Geometry check sheet. Reference: the model listing, model coordinates, mm. Face numbers are marked on the shaded views. A direction names the side the tool comes from. Give positions to 0.01 mm unless a question says otherwise; leave off trailing zeros. Order: outer loops, then holes, each group sorted by start corner. A loop starts at its lowest first (then second) coordinate and runs counter-clockwise, first axis right, second up.
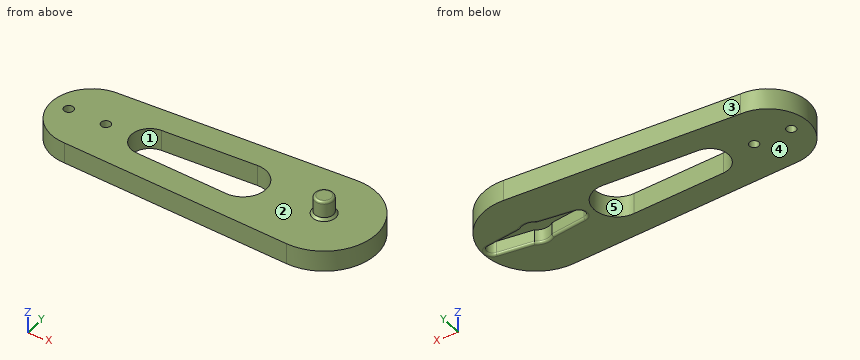
```python
from build123d import *

# Parameters (mm, degrees)
BOSS_EXTRUDE1_DEPTH = 9
BOSS_EXTRUDE2_START = 9
SKETCH3_R           = 4
BOSS_EXTRUDE2_DEPTH = 8
FILLET1_R           = 1
CHAMFER2_SIZE       = 1
CUT_EXTRUDE1_DEPTH  = 6
FILLET3_R           = 1
SKETCH6_R           = 2.05
CUT_EXTRUDE2_DEPTH  = 10


with BuildPart() as part:
    # Sketch2 → Boss-Extrude1 (new body)
    with BuildSketch(Plane(origin=(0, 0, 0), x_dir=(0, 1, 0), z_dir=(0, 0, 1))):
        with BuildLine():
            Line((22.471608109, 1.129968581), (17.5, 100))
            ThreePointArc((17.5, 100), (0, 117.5), (-17.5, 100))
            Line((-17.5, 100), (-22.471608109, 1.129968581))
            ThreePointArc((-22.471608109, 1.129968581), (0, -22.5), (22.471608109, 1.129968581))
        make_face()
    extrude(amount=BOSS_EXTRUDE1_DEPTH)

    # Sketch3 → Boss-Extrude2 (add)
    with BuildSketch(Plane(origin=(0, 0, 0), x_dir=(0, 1, 0), z_dir=(0, 0, 1)).offset(BOSS_EXTRUDE2_START)):
        with Locations(Location((0, 0, 0), (0, 0, 270))):
            Circle(SKETCH3_R)
    extrude(amount=BOSS_EXTRUDE2_DEPTH)

    # Fillet1
    fillet1_edges = [part.edges().sort_by_distance(p)[0] for p in [
        (-4, 0, 17),
    ]]
    fillet(fillet1_edges, radius=FILLET1_R)

    # Chamfer2
    chamfer2_edges = [part.edges().sort_by_distance(p)[0] for p in [
        (-4, 0, 9),
    ]]
    chamfer(chamfer2_edges, length=CHAMFER2_SIZE)

    # Sketch5 → Cut-Extrude1 (cut)
    with BuildSketch(Plane(origin=(0, 0, 0), x_dir=(0, 1, 0), z_dir=(0, 0, 1))):
        with BuildLine():
            Line((-2.677123133, -18.850730282), (-4.65, -3.791767398))
            ThreePointArc((-4.65, -3.791767398), (-6, 0), (-4.65, 3.791767398))
            Line((-4.65, 3.791767398), (-2.677123133, 18.850730282))
            ThreePointArc((-2.677123133, 18.850730282), (0, 21.2), (2.677123133, 18.850730282))
            Line((2.677123133, 18.850730282), (4.65, 3.791767398))
            ThreePointArc((4.65, 3.791767398), (6, 0), (4.65, -3.791767398))
            Line((4.65, -3.791767398), (2.677123133, -18.850730282))
            ThreePointArc((2.677123133, -18.850730282), (0, -21.2), (-2.677123133, -18.850730282))
        make_face()
    extrude(amount=CUT_EXTRUDE1_DEPTH, mode=Mode.SUBTRACT)

    # Fillet3
    fillet3_edges = [part.edges().sort_by_distance(p)[0] for p in [
        (-21.2, 0, 0),
        (0, -6, 0),
        (21.2, 0, 0),
        (0, 6, 0),
        (-11.32124884, 3.663561567, 0),
        (11.32124884, 3.663561567, 0),
        (11.32124884, -3.663561567, 0),
        (-11.32124884, -3.663561567, 0),
    ]]
    fillet(fillet3_edges, radius=FILLET3_R)

    # Sketch6 → Cut-Extrude2 (cut)
    with BuildSketch(Plane(origin=(0, 0, 0), x_dir=(0, 1, 0), z_dir=(0, 0, 1))):
        with Locations(Location((0, 110, 0), (0, 0, 270))):
            Circle(SKETCH6_R)
        with Locations(Location((0, 94, 0), (0, 0, 270))):
            Circle(SKETCH6_R)
        with BuildLine():
            Line((-7.989993742, 75.4), (-9.987492178, 35.5))
            ThreePointArc((-9.987492178, 35.5), (0, 25), (9.987492178, 35.5))
            Line((9.987492178, 35.5), (7.989993742, 75.4))
            ThreePointArc((7.989993742, 75.4), (0, 83), (-7.989993742, 75.4))
        make_face()
    extrude(amount=CUT_EXTRUDE2_DEPTH, mode=Mode.SUBTRACT)


solid = part.part
```
Q1. Cross-section at A-A, the plane z = 3.75. Record the boundary of the cut face in (x, y).
Q2. Access from +Z, -Z, +X, -X, +Y, -Y to the whole of each face (thin tool, end or side, straight path). Record for the marked faces 4 and 5.
Q3. Thickness scan on L1, parallel to X at y = 0, z = 3.5; L2, parallel to X at y = 0, z = 7.25; L3, parallel to Z at x = -58, y = 14. Record the ranges inside material, lowest first.
Q4. Cross-section at D-D, the plane x = -78. Record the boundary of the cut face in (y, z), and give its area (3 significant figures).
Q5. Release check for a two-part mould opening along Y. For the marked faces 1, 2 and 3 record: pulls with the +Y half, pulls with the -Y half, needs draft (parallel to the pull), parting line crosses it, or undercut.
Q6. Cross-section at C-C, the plane z = 12.25. Record the boundary of the cut face in (x, y), and give its area (3 significant figures).
Q7. Gauge pin test, flat ends, axial feed: P1, Ø3, axis at x = 3, z = 2.5, coming from the -Y side; P2, Ø5, axis at x = -12, z = 13.5, coming from the -Y side; P3, Ø8, axis at y = 7, z = 6, coming from the +X side; P4, Ø10, axis at x = -1.5, y = -9, coming from the -Z side. Record the tip position at first contact, or that the pin passes through.
Q8. Cross-section at B-B, the plane x = -110. Record the boundary of the cut face in (y, z), and give its area (3 significant figures).
Answers follow:
1. outline: (-100, -17.5) - (-1.13, -22.47) arc R22.5 ccw (long way) to (-1.13, 22.47) - (-100, 17.5) arc R17.5 ccw to start; hole circle Ø4.1 at (-110, 0); hole circle Ø4.1 at (-94, 0); hole (-75.4, -7.99) - (-35.5, -9.99) arc R10 ccw (long way) to (-35.5, 9.99) - (-75.4, 7.99) arc R8 ccw to start; hole (-18.85, -2.68) - (-3.79, -4.65) arc R6 ccw to (3.79, -4.65) - (18.85, -2.68) arc R2.7 ccw to (18.85, 2.68) - (3.79, 4.65) arc R6 ccw to (-3.79, 4.65) - (-18.85, 2.68) arc R2.7 ccw to start
2. face 4: -Z, +X, -X, +Y, -Y
2. face 5: +Z, -Z
3. L1: x = -117.5 to -112.05, -107.95 to -96.05, -91.95 to -83, -25 to -21.2, 21.2 to 22.5
3. L2: x = -117.5 to -112.05, -107.95 to -96.05, -91.95 to -83, -25 to 22.5
3. L3: z = 0 to 9
4. outline: (-18.61, 0) - (-7.42, 0) - (-7.42, 9) - (-18.61, 9) - close; (7.42, 0) - (18.61, 0) - (18.61, 9) - (7.42, 9) - close
4. area: 201 mm2
5. face 1: undercut
5. face 2: needs draft
5. face 3: pulls with the +Y half
6. outline: circle Ø8 at (0, 0)
6. area: 50.3 mm2
7. P1: stops at y = -22.45
7. P2: passes through
7. P3: stops at x = 22.3
7. P4: stops at z = 0
8. outline: (-14.36, 0) - (-2.05, 0) - (-2.05, 9) - (-14.36, 9) - close; (2.05, 0) - (14.36, 0) - (14.36, 9) - (2.05, 9) - close
8. area: 222 mm2
